CAD build for the part. Positions are in the model's coordinates, mm. Face numbers are marked on the shaded views. Round coordinates to 2 decimals unless told otherwise and drop trailing zeros. Order: outer loops, then holes, each group sorted by start corner. A loop starts at its lowest first (then second) coordinate and runs counter-clockwise, first axis right, second up. Notation, with made-up numbers: (73.25, 26.5) - (101.25, 26.5) arc R18 ccw to (101.25, 43.5) - close; hole circle Ø8 at (-13, 55). An arc over 180 degrees is marked (long way). Use one line per item in the form item = value. Start each with the question number.
from build123d import *

# Parameters (mm, degrees)
F1_ANGLE = 180
F2_R     = 0.1778


with BuildPart() as f1:
    # F0 (on Front) → F1 (revolve)
    with BuildSketch(Plane.XZ):
        with BuildLine():
            Line((3.556, 13.974021), (3.556, 2.431545))
            Line((3.556, 2.431545), (2.904469, 0))
            Line((2.904469, 0), (2.286, 0))
            Line((2.286, 0), (2.286, -0.381))
            Line((2.286, -0.381), (3.196821, -0.381))
            Line((3.196821, -0.381), (3.937, 2.381385))
            Line((3.937, 2.381385), (3.937, 13.980661))
            ThreePointArc((3.937, 13.980661), (2.775962, 23.630641), (0, 32.945369))
            Line((0, 32.945369), (0, 31.880476))
            ThreePointArc((0, 31.880476), (2.500884, 23.070804), (3.556, 13.974021))
        make_face()
    revolve(axis=Axis((0, 0, 32.412922), (0, 0, 1)), revolution_arc=F1_ANGLE)

    # F2
    f2_edges = [f1.edges().sort_by_distance(p)[0] for p in [
        (0, 2.286, 0),
        (0, 2.286, -0.381),
        (0, 3.196821, -0.381),
    ]]
    fillet(f2_edges, radius=F2_R)


solid = f1.part
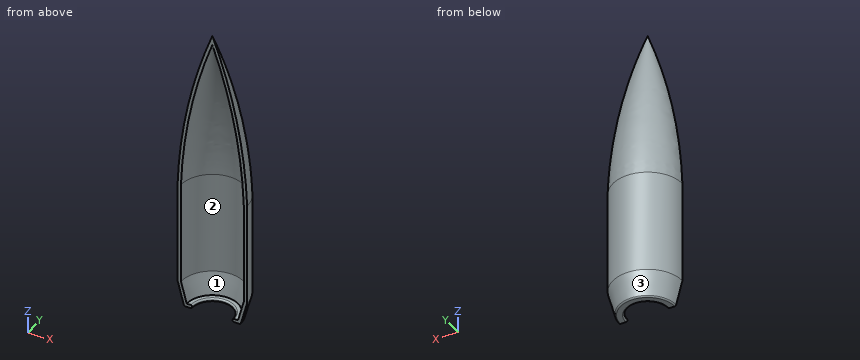
(1) Mould opens along X. For the marked faces 1, 2 and 3 say: pulls with the +X half, pulls with the -X half, needs draft (parallel to the pull), parting line crosses it, or undercut.
(2) Flat gauge pins, fed straight in: P1, Ø1, axis at y = 3, z = 5.5, coming from the +X side; P2, Ø4, axis at x = 2.5, z = 19.5, coming from the +Y side. Where does each tip first touch, or does it go through?
(3) Slice it at A-A (z = 10). Give the cut face in (x, y).
(4) Wall check: line 1 (X direction, y = 0.6, z = 29.5); line 2 (X direction, y = 2.3, z = 1) (3 decimals); line 3 (Y direction, x = -1.25, z = 8). Give the ranges that are in metal, low to high. Write a range as [from, to].
Results list:
q1.face_1 = undercut
q1.face_2 = undercut
q1.face_3 = parting line crosses it
q2.P1 = 3.04
q2.P2 = 3.52
q3.outline = (-3.94, 0) - (-3.56, 0) arc R3.56 cw to (3.56, 0) - (3.94, 0) arc R3.94 ccw to start
q4.line_1 = [-1.07, -0.57], [0.57, 1.07]
q4.line_2 = [-2.726, -2.185], [2.185, 2.726]
q4.line_3 = [3.33, 3.73]
